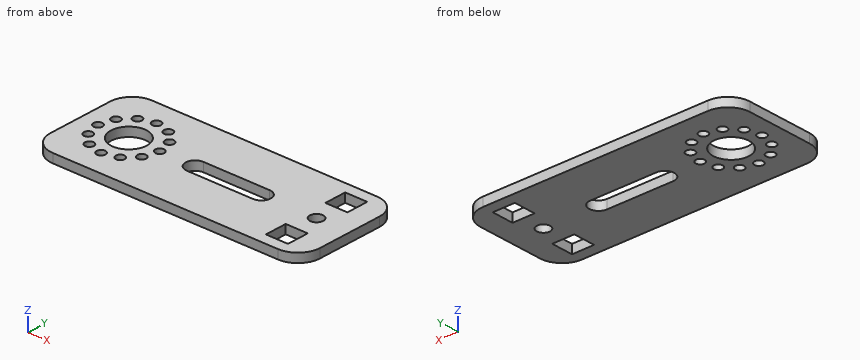
```python
from build123d import *

# Parameters (mm, degrees)
BOSS_EXTRU_1_START       = -2
BOSS_EXTRU_1_OUTLINE_W   = 61
BOSS_EXTRU_1_OUTLINE_H   = 25
BOSS_EXTRU_1_OUTLINE_W_2 = 5
BOSS_EXTRU_1_OUTLINE_H_2 = 5
BOSS_EXTRU_1_OUTLINE_R   = 1
BOSS_EXTRU_1_OUTLINE_R_2 = 1.5
BOSS_EXTRU_1_OUTLINE_R_3 = 4.05
BOSS_EXTRU_1_DEPTH       = 2
CONG_1_R                 = 5


# Read off the part's stored shape, not the designer's step: Boss.-Extru.1
with BuildPart() as part:
    # Boss.-Extru.1 outline → Boss.-Extru.1 (new body)
    with BuildSketch(Plane(origin=(0, 0, 0), x_dir=(-1, 0, 0), z_dir=(0, 0, -1)).offset(BOSS_EXTRU_1_START)):
        with Locations((-30.5, 0)):
            Rectangle(BOSS_EXTRU_1_OUTLINE_W, BOSS_EXTRU_1_OUTLINE_H)
        with Locations((-53.5, -7.5)):
            Rectangle(BOSS_EXTRU_1_OUTLINE_W_2, BOSS_EXTRU_1_OUTLINE_H_2, mode=Mode.SUBTRACT)
        with Locations((-11, -7)):
            Circle(BOSS_EXTRU_1_OUTLINE_R, mode=Mode.SUBTRACT)
        with Locations((-17.062177826, -3.5)):
            Circle(BOSS_EXTRU_1_OUTLINE_R, mode=Mode.SUBTRACT)
        with Locations((-14.5, -6.062177826)):
            Circle(BOSS_EXTRU_1_OUTLINE_R, mode=Mode.SUBTRACT)
        with Locations((-7.5, -6.062177826)):
            Circle(BOSS_EXTRU_1_OUTLINE_R, mode=Mode.SUBTRACT)
        with Locations((-4.937822174, -3.5)):
            Circle(BOSS_EXTRU_1_OUTLINE_R, mode=Mode.SUBTRACT)
        with Locations((-53.5, 0)):
            Circle(BOSS_EXTRU_1_OUTLINE_R_2, mode=Mode.SUBTRACT)
        with BuildLine():
            ThreePointArc((-26, 2.1), (-23.9, 0), (-26, -2.1))
            Line((-26, -2.1), (-41, -2.1))
            ThreePointArc((-41, -2.1), (-43.1, 0), (-41, 2.1))
            Line((-41, 2.1), (-26, 2.1))
        make_face(mode=Mode.SUBTRACT)
        with Locations((-53.5, 7.5)):
            Rectangle(BOSS_EXTRU_1_OUTLINE_W_2, BOSS_EXTRU_1_OUTLINE_H_2, mode=Mode.SUBTRACT)
        with Locations((-18, 0)):
            Circle(BOSS_EXTRU_1_OUTLINE_R, mode=Mode.SUBTRACT)
        with Locations((-17.062177826, 3.5)):
            Circle(BOSS_EXTRU_1_OUTLINE_R, mode=Mode.SUBTRACT)
        with Locations((-11, 0)):
            Circle(BOSS_EXTRU_1_OUTLINE_R_3, mode=Mode.SUBTRACT)
        with Locations((-4, 0)):
            Circle(BOSS_EXTRU_1_OUTLINE_R, mode=Mode.SUBTRACT)
        with Locations((-14.5, 6.062177826)):
            Circle(BOSS_EXTRU_1_OUTLINE_R, mode=Mode.SUBTRACT)
        with Locations((-4.937822174, 3.5)):
            Circle(BOSS_EXTRU_1_OUTLINE_R, mode=Mode.SUBTRACT)
        with Locations((-7.5, 6.062177826)):
            Circle(BOSS_EXTRU_1_OUTLINE_R, mode=Mode.SUBTRACT)
        with Locations((-11, 7)):
            Circle(BOSS_EXTRU_1_OUTLINE_R, mode=Mode.SUBTRACT)
    extrude(amount=BOSS_EXTRU_1_DEPTH)

    # Congé1
    cong_1_edges = [part.edges().sort_by_distance(p)[0] for p in [
        (61, 12.5, 1),
        (0, 12.5, 1),
        (0, -12.5, 1),
        (61, -12.5, 1),
    ]]
    fillet(cong_1_edges, radius=CONG_1_R)


solid = part.part
```
CAD build for the part. Positions are in the model's coordinates, mm. Round coordinates to 2 decimals unless told otherwise and drop trailing zeros. Order: outer loops, then holes, each group sorted by start corner. A loop starts at its lowest first (then second) coordinate and runs counter-clockwise, first axis right, second up.
Item 1: Saw through at C-C on z = 1.45. State how many separate pieces and enclosed holes the cut face has, then the cut area to 3 significant figures.
Item 2: Saw through at B-B on x = 37.5. Write the cut outline in (y, z).
Item 3: Saw through at A-A on y = 0. Write the cut outline in (x, z).
Item 4: Probe line 1 along Y through (x, z) = (29, 0.8); line 2 along X through (y, z) = (5.25, 0.4); line 3 along X through (y, z) = (6.75, 1.75). List the from-to ranges inside material, lowest first.
Item 5: Pin check, flat tip, straight feed: pin 1 (1 mm diameter, centred on y = 9.5, z = 1.5, fed in from +X). Stop position of the tip, or through.
Item 6: Saw through at D-D on y = -3.5. Write the cut outline in (x, z).
Reported:
1. separate pieces: 1
1. enclosed holes: 17
1. area: 1,280 mm2
2. outline: (-12.5, 0) - (-2.1, 0) - (-2.1, 2) - (-12.5, 2) - close; (2.1, 0) - (12.5, 0) - (12.5, 2) - (2.1, 2) - close
3. outline: (0, 0) - (3, 0) - (3, 2) - (0, 2) - close; (5, 0) - (6.95, 0) - (6.95, 2) - (5, 2) - close; (15.05, 0) - (17, 0) - (17, 2) - (15.05, 2) - close; (19, 0) - (23.9, 0) - (23.9, 2) - (19, 2) - close; (43.1, 0) - (52, 0) - (52, 2) - (43.1, 2) - close; (55, 0) - (61, 0) - (61, 2) - (55, 2) - close
4. line 1: y = -12.5 to -2.1, 2.1 to 12.5
4. line 2: x = 0 to 6.92, 8.08 to 13.92, 15.08 to 51, 56 to 61
4. line 3: x = 0 to 6.77, 8.23 to 10.03, 11.97 to 13.77, 15.23 to 51, 56 to 61
5. pin 1: stops at x = 60.77
6. outline: (0, 0) - (3.94, 0) - (3.94, 2) - (0, 2) - close; (5.94, 0) - (8.96, 0) - (8.96, 2) - (5.94, 2) - close; (13.04, 0) - (16.06, 0) - (16.06, 2) - (13.04, 2) - close; (18.06, 0) - (61, 0) - (61, 2) - (18.06, 2) - close
